Autodesk Inventor part; units mm, degrees
ref_plane "YZ Plane" through (0, 0, 0) normal (1, 0, 0) x (0, 1, 0)
ref_plane "XZ Plane" through (0, 0, 0) normal (0, 1, 0) x (-1, 0, 0)
ref_plane "XY Plane" through (0, 0, 0) normal (0, 0, 1) x (1, 0, 0)
sketch "Sketch1" plane through (0, 0, 0) normal (0, 0, 1) x (1, 0, 0)
  line L0 (6, -6) -> (-6, -6)
  line L1 (-6, -6) -> (-6, 6)
  line L2 (-6, 6) -> (6, 6)
  line L3 (6, 6) -> (6, -6)
  point P0 (0, 0)
  point P1 (0, 0)
  dimension "d0" = 12
  dimension "d1" = 12
  dimension "d2" = 6
  dimension "d3" = 6
extrude "Extrusion1" add sketch "Sketch1" along normal blind 4
fillet "Fillet1" radius 2 4 edges at (-6, 6, 2) (-6, -6, 2) (6, 6, 2) (6, -6, 2)
sketch "Sketch2" plane through (0, 0, 4) normal (0, 0, 1) x (1, 0, 0)
  circle A0 centre (0, 0) radius 3.5
  dimension "d7" = 7
extrude "Extrusion2" add sketch "Sketch2" along normal blind 4
fillet "Fillet2" radius 0.5 1 edges at (-3.5, 0, 8)
properties part number "Button" material "PET Plastic"
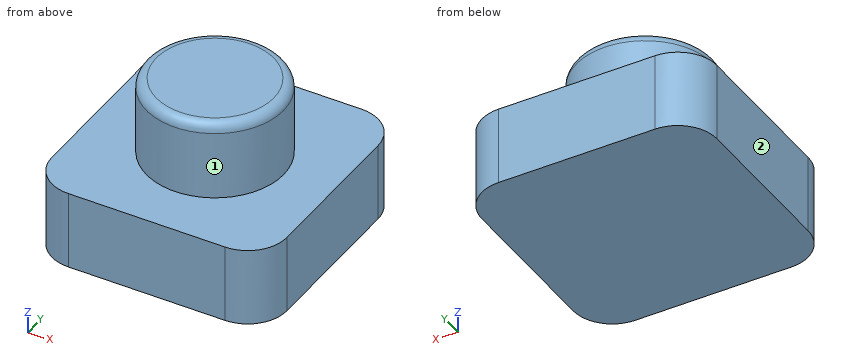
The listing builds one solid part. Answer for the finished solid, in the listing's coordinates (mm). Face numbers are marked on the shaded views. A direction names the side the tool comes from. Round coordinates to 2 decimals unless told otherwise and drop trailing zeros. Loops run counter-clockwise (first coordinate to the right, second up) from the corner with the lowest first, then second, coordinate; pieces in that order, holes last.
1) A cutting plane is placed at C-C on z = 0.5. Determine the outline of the cut face in (x, y), plus the area to 3 significant figures.
Outcome:
outline: (-6, -4) arc R2 ccw to (-4, -6) - (4, -6) arc R2 ccw to (6, -4) - (6, 4) arc R2 ccw to (4, 6) - (-4, 6) arc R2 ccw to (-6, 4) - close
area: 141 mm2
2) A cutting plane is placed at A-A on x = 0. Determine the outline of the cut face in (y, z), plus the area to 3 significant figures.
Outcome:
outline: (-6, 0) - (6, 0) - (6, 4) - (3.5, 4) - (3.5, 7.5) arc R0.5 ccw to (3, 8) - (-3, 8) arc R0.5 ccw to (-3.5, 7.5) - (-3.5, 4) - (-6, 4) - close
area: 75.9 mm2
3) Consider line 1 (Z direction, x = 5.5, y = 0.25); line 2 (Y direction, x = 3, z = 5.5); line 3 (Y direction, x = 5.5, z = 2.5). Determine where each line is inside the solid, lowest interval first.
Outcome:
line 1: z = 0 to 4
line 2: y = -1.8 to 1.8
line 3: y = -5.32 to 5.32
4) For the marked faces 1 and 2, determine the directions among +Z, -Z, +X, -X, +Y, -Y from which every point of the face is accessible in a straight line to the end or side of a thin tool.
Outcome:
face 1: +Z
face 2: +Z, -Z, -X, +Y, -Y
5) A cutting plane is placed at D-D on z = 5.5. Determine the outline of the cut face in (x, y), plus the area to 3 significant figures.
Outcome:
outline: circle Ø7 at (0, 0)
area: 38.5 mm2
